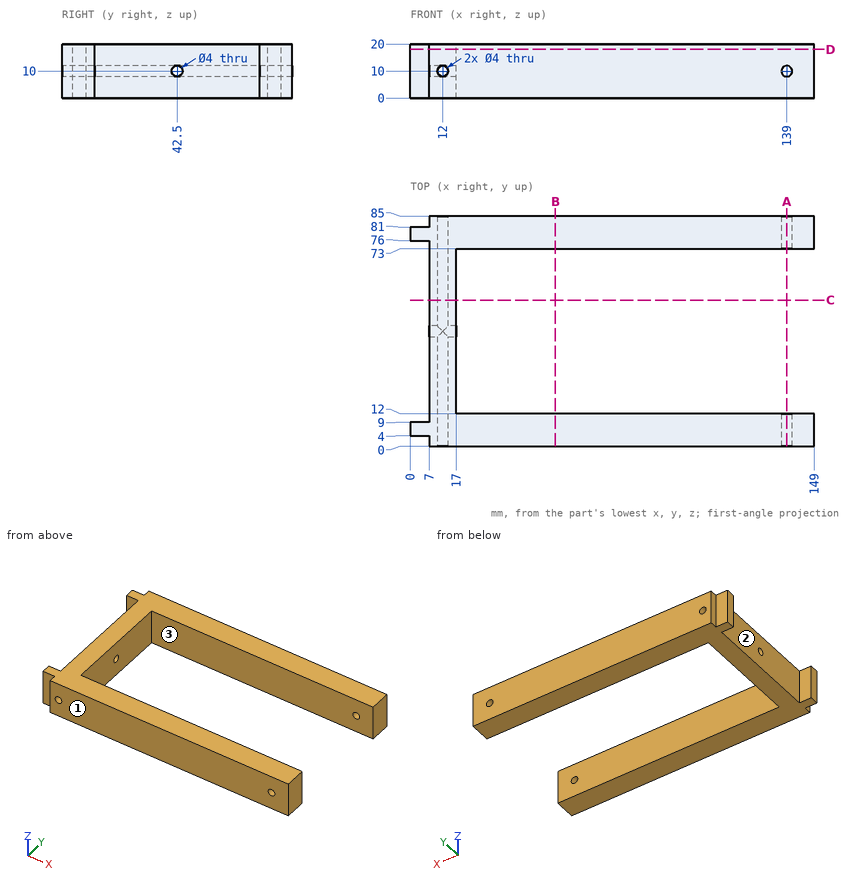
Study the drawing (mm; zero at the part's minimum x, y, z) and answer. A direction names the side the tool comes from. Give positions to 0.01 mm unless a question says otherwise; leave off trailing zeros. Loops run counter-clockwise (first coordinate to the right, second up) from the corner with the lowest first, then second, coordinate; pieces in that order, holes last. Notation, with made-up numbers: (5.5, -5.5) - (62.5, -5.5) arc R26 ccw to (62.5, 19.5) - close; hole circle Ø6 at (33.25, -13.75). An arc over 180 degrees is marked (long way). Return JSON: item names as keys, results as strings. Group by question number.
1. Find section B-B (x = 53.5). Write down the section's boundary in (y, z).
2. Straight lines are drawn through the part: line 1 (Z direction, x = 10.95, y = 42.5); line 2 (Y direction, x = 121.5, z = 14.5); line 3 (X direction, y = 38, z = 9.75). For each, find the intervals that lie inside material, in ascending order. Write a range as [from, to].
3. Find section D-D (z = 18). Write down the section's boundary in (x, y), then the cut area to 3 significant figures.
4. Find section A-A (x = 139). Write down the section's boundary in (y, z).
5. Find section C-C (y = 54). Write down the section's boundary in (x, z).
6. Given pin 1 Ø4.5 at (y, z) = (83.5, 13) entering from -X; pin 2 Ø6 at (y, z) = (42, 6) entering from +X; pin 3 Ø6.5 at (x, z) = (139, 10) entering from -Y; pin 4 Ø7.5 at (x, z) = (3, 14) entering from -Y, each flat-ended and moving along its own axis, determine where each tip first touches the part or whether it passes through.
7. Which of the six approach directions +Z, -Z, +X, -X, +Y, -Y give full straight-line access (tool end or side, diameter ignored) to the marked faces 1, 2 and 3?
Verdict:
{
 "1": {"outline": "(0, 0) - (12, 0) - (12, 20) - (0, 20) - close; (73, 0) - (85, 0) - (85, 20) - (73, 20) - close"},
 "2": {"line 1": "z = [0, 8], [12, 20]", "line 2": "y = [0, 12], [73, 85]", "line 3": "x = [7, 10.02], [13.98, 17]"},
 "3": {"outline": "(0, 4) - (7, 4) - (7, 0) - (149, 0) - (149, 12) - (17, 12) - (17, 73) - (149, 73) - (149, 85) - (7, 85) - (7, 81) - (0, 81) - (0, 76) - (7, 76) - (7, 9) - (0, 9) - close", "area": "4,090 mm^2"},
 "4": {"outline": "(0, 0) - (12, 0) - (12, 8) - (0, 8) - close; (0, 12) - (12, 12) - (12, 20) - (0, 20) - close; (73, 0) - (85, 0) - (85, 8) - (73, 8) - close; (73, 12) - (85, 12) - (85, 20) - (73, 20) - close"},
 "5": {"outline": "(7, 0) - (17, 0) - (17, 20) - (7, 20) - close; hole circle Ø4 at (12, 10)"},
 "6": {"pin 1": "stops at x = 7", "pin 2": "stops at x = 17", "pin 3": "stops at y = 0", "pin 4": "stops at y = 4"},
 "7": {"face 1": "+Z, -Z, +X, -X, -Y", "face 2": "+Z, -Z, -X", "face 3": "+Z, -Z, +X"}
}
